```python
from build123d import *

# Parameters (mm, degrees)
SKETCH1_W           = 127
SKETCH1_H           = 3.175
BOSS_EXTRUDE2_DEPTH = 110.236
SKETCH2_R           = 2.286
SKETCH2_R_2         = 9.5123
BOSS_EXTRUDE3_DEPTH = 3.175
SKETCH3_R           = 2.54
CUT_EXTRUDE1_DEPTH  = 4.175


with BuildPart() as part:
    # Sketch1 → Boss-Extrude2 (new body)
    with BuildSketch(Plane.XY):
        with BuildLine():
            Line((-35.3822, 0), (-32.2072, 0))
            ThreePointArc((-32.2072, 0), (0, -32.2072), (32.2072, 0))
            Line((32.2072, 0), (35.3822, 0))
            ThreePointArc((35.3822, 0), (0, -35.3822), (-35.3822, 0))
        make_face()
        with Locations((0, -33.7947)):
            Rectangle(SKETCH1_W, SKETCH1_H)
    extrude(amount=BOSS_EXTRUDE2_DEPTH)

    # Sketch2 → Boss-Extrude3 (add)
    with BuildSketch(Plane.XY.offset(110.236)):
        Polygon((-35.3822, -35.3822), (35.3822, -35.3822), (63.5, -35.3822), (63.5, -32.2072), (35.3822, -32.2072), (35.3822, 35.4838), (-35.3822, 35.4838), (-35.3822, -32.2072), (-63.5, -32.2072), (-63.5, -35.3822), align=None)
        with Locations((-25.146, 0)):
            Circle(SKETCH2_R, mode=Mode.SUBTRACT)
        with Locations((0, 25.146)):
            Circle(SKETCH2_R, mode=Mode.SUBTRACT)
        with Locations((25.146, 0)):
            Circle(SKETCH2_R, mode=Mode.SUBTRACT)
        with Locations((0, -25.146)):
            Circle(SKETCH2_R, mode=Mode.SUBTRACT)
        Circle(SKETCH2_R_2, mode=Mode.SUBTRACT)
    extrude(amount=BOSS_EXTRUDE3_DEPTH)

    # Sketch3 → Cut-Extrude1 (cut, through all)
    with BuildSketch(Plane(origin=(0, -32.2072, 0), x_dir=(1, 0, 0), z_dir=(0, 1, 0))):
        with Locations((49.403, -85.09)):
            Circle(SKETCH3_R)
        with Locations((49.403, -28.321)):
            Circle(SKETCH3_R)
        with Locations((-49.403, -85.09)):
            Circle(SKETCH3_R)
        with Locations((-49.403, -28.321)):
            Circle(SKETCH3_R)
    extrude(amount=-CUT_EXTRUDE1_DEPTH, mode=Mode.SUBTRACT)


solid = part.part
```
Model file for the job. Use its own axes, mm. A direction names the side the tool comes from. Coordinates: 2 decimals unless noted, no trailing zeros. Write each loop counter-clockwise with the first axis right and the second up, starting at its lowest first coordinate (ties: lowest second). Pieces come first, ordered by that corner, then holes. Notation, with made-up numbers: (21, -2.75) - (59, -2.75) arc R21 ccw to (59, 4.25) - close; hole circle Ø6 at (5, -0.75). An arc over 180 degrees is marked (long way). Use a Markdown table: item, result. Add a question column.
Item 1: Drill centre lines: line 1 along X through (y, z) = (-34.5, 85.09); line 2 along Y through (x, z) = (0, 111.1); line 3 along Y through (x, z) = (51, 88). Where is each one in solid material? Low to high.
Item 2: Band-saw the part on C-C, the plane y = -5.5. Write the cut outline in (x, z), and give its area (3 significant figures).
Item 3: 3-axis set-ups, long thin cutter, end or side, ignore diameter. For faces 1 (the face through (0.7, -32.2, 54.3)), 2 (the face through (-30, -24, 110.236)), 3 (the face through (-35.382, 2, 112)), 4 (the face through (39, -32.207, 56)), 5 (the face through (35.382, 1, 112)): which of +Z, -Z, +X, -X, +Y, -Y reach the whole face in a straight line?
Item 4: Band-saw the part on A-A, the plane x = 0. Write the cut outline in (y, z), and give its area (3 significant figures).
Item 5: Drop flat-ended pins along their axis: pin 1 (3 mm diameter, centred on x = -46, z = 83, fed in from +Y); pin 2 (1 mm diameter, centred on y = 12.5, z = 112, fed in from -X); pin 3 (6.5 mm diameter, centred on x = -49.403, z = 85.09, fed in from -Y); pin 4 (1 mm diameter, centred on y = 2.5, z = 111.5, fed in from +X). Give the stop position or say it passes through.
Item 6: Band-saw the part on D-D, the plane y = -16. Write the cut outline in (x, z), and give its area (3 significant figures).
Item 7: Two-plate mould, pull along Z, no slides. Class faces 6 (the face through (0, -33, 0)), 7 (the face through (47.531, -33.772, 26.604)), 8 (the face through (-15, 1, 113.411)): pulls with the +Z half, pulls with the -Z half, needs draft (parallel to the pull), parting line crosses it, or undercut.
Item 8: Band-saw the part on B-B, the plane z = 74. Write the cut outline in (x, y).
A:
| question | item | result |
|---|---|---|
| 1 | line 1 | x = -63.5 to -51.94, -46.86 to 46.86, 51.94 to 63.5 |
| 1 | line 2 | y = -35.38 to -27.43, -22.86 to -9.51, 9.51 to 22.86, 27.43 to 35.48 |
| 1 | line 3 | y = -35.38 to -32.21 |
| 2 | outline | (-35.38, 110.24) - (-34.95, 110.24) - (-34.95, 0) - (-31.73, 0) - (-31.73, 110.24) - (-7.76, 110.24) - (-7.76, 113.41) - (-35.38, 113.41) - close; (7.76, 110.24) - (31.73, 110.24) - (31.73, 0) - (34.95, 0) - (34.95, 110.24) - (35.38, 110.24) - (35.38, 113.41) - (7.76, 113.41) - close |
| 2 | area | 885 mm² |
| 3 | face 1 | -Z, +Y |
| 3 | face 2 | -Z, -X |
| 3 | face 3 | +Z, -Z, -X, +Y |
| 3 | face 4 | -Z, +X |
| 3 | face 5 | +Z, -Z, +X, +Y |
| 4 | outline | (-35.38, 0) - (-32.21, 0) - (-32.21, 110.24) - (-27.43, 110.24) - (-27.43, 113.41) - (-35.38, 113.41) - close; (-22.86, 110.24) - (-9.51, 110.24) - (-9.51, 113.41) - (-22.86, 113.41) - close; (9.51, 110.24) - (22.86, 110.24) - (22.86, 113.41) - (9.51, 113.41) - close; (27.43, 110.24) - (35.48, 110.24) - (35.48, 113.41) - (27.43, 113.41) - close |
| 4 | area | 486 mm² |
| 5 | pin 1 | stops at y = -32.21 |
| 5 | pin 2 | stops at x = -35.38 |
| 5 | pin 3 | stops at y = -35.38 |
| 5 | pin 4 | stops at x = 35.38 |
| 6 | outline | (-35.38, 110.24) - (-31.56, 110.24) - (-31.56, 0) - (-27.95, 0) - (-27.95, 110.24) - (27.95, 110.24) - (27.95, 0) - (31.56, 0) - (31.56, 110.24) - (35.38, 110.24) - (35.38, 113.41) - (-35.38, 113.41) - close |
| 6 | area | 1,020 mm² |
| 7 | face 6 | pulls with the -Z half |
| 7 | face 7 | undercut |
| 7 | face 8 | pulls with the +Z half |
| 8 | outline | (-63.5, -35.38) - (63.5, -35.38) - (63.5, -32.21) - (14.65, -32.21) arc R35.38 ccw to (35.38, 0) - (32.21, 0) arc R32.21 cw to (-32.21, 0) - (-35.38, 0) arc R35.38 ccw to (-14.65, -32.21) - (-63.5, -32.21) - close |
